from build123d import *

# Parameters (mm, degrees)
F0_W     = 68.072
F0_H     = 82.042
F1_DEPTH = 1.524
F3_D     = 2.7051
F4_R     = 11.303
F5_DEPTH = 1.525


with BuildPart() as f1:
    # F0 (on Front) → F1 (new body)
    with BuildSketch(Plane.XZ):
        with Locations((34.036, -41.021)):
            Rectangle(F0_W, F0_H)
    extrude(amount=F1_DEPTH)

    # F3 (through all)
    with Locations(Plane.XZ.offset(1.524)):
        with Locations((6.096, -5.969), (61.976, -5.969), (61.976, -76.073), (6.096, -76.073)):
            Hole(F3_D / 2)

    # F4 (on face) → F5 (cut, through all)
    with BuildSketch(Plane.XZ.offset(1.524)):
        with Locations((34.036, -41.021)):
            Circle(F4_R)
    extrude(amount=-F5_DEPTH, mode=Mode.SUBTRACT)


solid = f1.part
Verification items for the finished model (mm, model axes). Give positions to 0.01 mm unless a question says otherwise; leave off trailing zeros. Write each loop counter-clockwise with the first axis right and the second up, starting at its lowest first coordinate (ties: lowest second). Pieces come first, ordered by that corner, then holes. Notation, with made-up numbers: M -25.75,82 L 22.25,82 A22 cw 22.25,95 Z; hole C -31,76 d3. An arc over 180 degrees is marked long. Write item = value, one per line.
(1) Draft check along X on faces 1 (the face through (6.389, -0.751, -77.393)), 2 (the face through (62.269, -0.751, -77.393)), 3 (the face through (26, 0, -31)). Enter one of: released by +X, released by -X, zero draft, split by the parting line, or undercut.
Found:
face_1 = undercut
face_2 = undercut
face_3 = zero draft
(2) Sectioned sample at D-D (y = -0.8). Record the cut outline in (x, z).
Found:
outline = M 0,-82.04 L 68.07,-82.04 L 68.07,0 L 0,0 Z; hole C 6.1,-76.07 d2.71; hole C 6.1,-5.97 d2.71; hole C 34.04,-41.02 d22.61; hole C 61.98,-76.07 d2.71; hole C 61.98,-5.97 d2.71
(3) Sectioned sample at B-B (z = -31). Record the cut outline in (x, y).
Found:
outline = M 0,-1.52 L 28.81,-1.52 L 28.81,0 L 0,0 Z; M 39.26,-1.52 L 68.07,-1.52 L 68.07,0 L 39.26,0 Z
(4) Sectioned sample at A-A (x = 61.5). Record the cut outline in (y, z), then the cut area to 3 significant figures.
Found:
outline = M -1.52,-82.04 L 0,-82.04 L 0,-77.34 L -1.52,-77.34 Z; M -1.52,-74.81 L 0,-74.81 L 0,-7.24 L -1.52,-7.24 Z; M -1.52,-4.7 L 0,-4.7 L 0,0 L -1.52,0 Z
area = 117 mm2
(5) Material ranges on line 1 (Z direction, x = 5, y = -0.6); line 2 (X direction, y = -0.9, z = -39.5); line 3 (X direction, y = -0.7, z = -7), recorded low to high.
Found:
line_1 = -82.04 to -76.87, -75.28 to -6.76, -5.18 to 0
line_2 = 0 to 22.84, 45.24 to 68.07
line_3 = 0 to 5.22, 6.97 to 61.1, 62.85 to 68.07
(6) Sectioned sample at C-C (x = 38.5). Record the cut outline in (y, z).
Found:
outline = M -1.52,-82.04 L 0,-82.04 L 0,-51.41 L -1.52,-51.41 Z; M -1.52,-30.64 L 0,-30.64 L 0,0 L -1.52,0 Z
